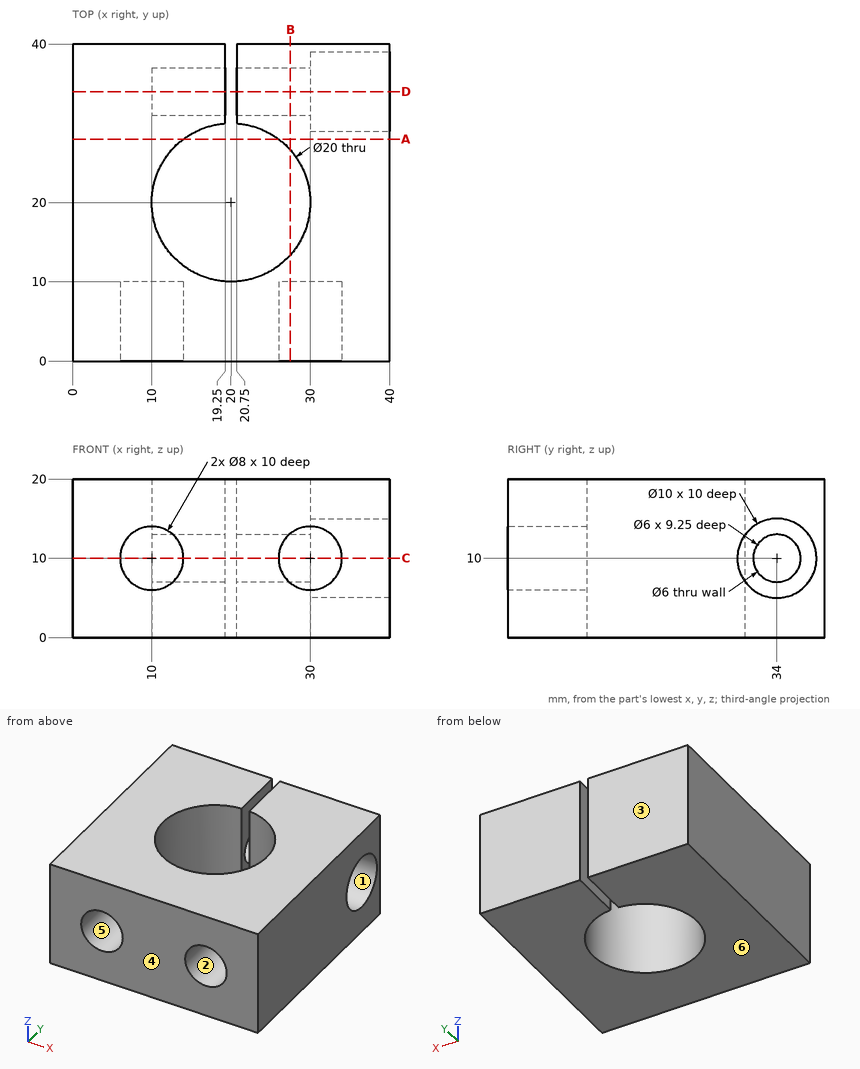
Geometry: see drawing. Coordinates: mm, zero at the bounding-box minimum. A direction names the side the tool comes from. Give positions to 0.01 mm unless a question says otherwise; leave off trailing zeros. Write each loop counter-clockwise with the first axis right and the second up, starting at its lowest first coordinate (ties: lowest second). Pieces come first, ordered by that corner, then holes. Notation, with made-up numbers: (9, -1.75) - (57, -1.75) arc R15 cw to (57, 11.25) - close; hole circle Ø11 at (45, 2.5). An arc over 180 degrees is marked (long way). Return JSON: item names as keys, results as strings. Group by question number.
1) Section D-D on y = 34. Return the cut outline in (x, z).
2) Set-up query: the marked faces 1, 2 and 3. Return all of +Z, -Z, +X, -X, +Y, -Y with unobstructed straight access to the full face (end or side cutting, diameter ignored); none if empty.
3) Line query: line 1 (Y direction, x = 12, z = 9.75); line 2 (X direction, y = 6.5, z = 10); line 3 (X direction, y = 28, z = 12). Output: solid intervals per line, ascending.
4) Section C-C on z = 10. Return the cut outline in (x, y).
5) Mould query, pull axis Z, two halves, no side actions, for the marked faces 4, 5 and 6. Classes: released by +Z, released by -Z, zero draft, split by the parting line, or undercut.
6) First-contact query: P1, Ø6.5, axis at y = 35, z = 9, coming from the +X side; P2, Ø4, axis at x = 31.5, z = 11, coming from the -Y side; P3, Ø5.5, axis at y = 34, z = 10, coming from the +X side. Flat tips, straight axial feed; report the tip coordinate or a pass-through.
7) Section B-B on x = 27.5. Return the cut outline in (y, z).
8) Section A-A on y = 28. Return the cut outline in (x, z).
Filled in:
{
 "1": {"outline": "(0, 0) - (19.25, 0) - (19.25, 7) - (10, 7) - (10, 13) - (19.25, 13) - (19.25, 20) - (0, 20) - close; (20.75, 0) - (40, 0) - (40, 5) - (30, 5) - (30, 7) - (20.75, 7) - close; (20.75, 13) - (30, 13) - (30, 15) - (40, 15) - (40, 20) - (20.75, 20) - close"},
 "2": {"face 1": "+X", "face 2": "-Y", "face 3": "+Z, -Z, +X, -X, +Y"},
 "3": {"line 1": "y = 10 to 14, 26 to 31.01, 36.99 to 40", "line 2": "x = 0 to 6, 14 to 26, 34 to 40", "line 3": "x = 0 to 14, 26 to 40"},
 "4": {"outline": "(0, 0) - (6, 0) - (6, 10) - (14, 10) - (14, 0) - (26, 0) - (26, 10) - (34, 10) - (34, 0) - (40, 0) - (40, 29) - (30, 29) - (30, 31) - (20.75, 31) - (20.75, 29.97) arc R10 cw (long way) to (19.25, 29.97) - (19.25, 31) - (10, 31) - (10, 37) - (19.25, 37) - (19.25, 40) - (0, 40) - close; (20.75, 37) - (30, 37) - (30, 39) - (40, 39) - (40, 40) - (20.75, 40) - close"},
 "5": {"face 4": "zero draft", "face 5": "undercut", "face 6": "released by -Z"},
 "6": {"P1": "stops at x = 30", "P2": "stops at y = 10", "P3": "stops at x = 10"},
 "7": {"outline": "(0, 0) - (13.39, 0) - (13.39, 20) - (0, 20) - (0, 13.12) - (10, 13.12) - (10, 6.88) - (0, 6.88) - close; (26.61, 0) - (40, 0) - (40, 20) - (26.61, 20) - close; hole circle Ø6 at (34, 10)"},
 "8": {"outline": "(0, 0) - (14, 0) - (14, 20) - (0, 20) - close; (26, 0) - (40, 0) - (40, 20) - (26, 20) - close"}
}
